Source: CAD feature listing. Evaluate the final solid. Frame: model axes, mm. Give positions to 0.01 mm unless a question says otherwise; leave off trailing zeros. Order: outer loops, then holes, each group sorted by start corner. A loop starts at its lowest first (then second) coordinate and runs counter-clockwise, first axis right, second up. Notation, with made-up numbers: M 43,74.5 L 100,74.5 A23 cw 100,85.5 Z; hole C -35.75,37 d7. An arc over 180 degrees is marked long. Use CSV: the item, a comma, the result in double quotes. Start each with the question number.
1. Pin query (flat end, axial travel): P1, Ø1, axis at x = -47, z = 1, coming from the +Y side; P2, Ø0.6, axis at x = -41.5, z = 1, coming from the -Y side. Return the tip coordinate at first contact, or that it passes through.
2. Section query C-C, the plane y = -3. Return the cut outline in (x, z), plus the area to 3 significant figures.
3. Line query: line 1 along Y through (x, z) = (1, 1.2); line 2 along X through (y, z) = (4.5, 0.85); line 3 along Y through (x, z) = (-22.5, 1.85). Output: solid intervals per line, ascending. Write a range as [from, to].
4. Section query A-A, the plane x = -2. Return the cut outline in (y, z), plus the area to 3 significant figures.
5. Section query D-D, the plane x = 40. Return the cut outline in (y, z), plus the area to 3 significant figures.
6. Section query B-B, the plane y = 15.5. Return the cut outline in (x, z).
from build123d import *

# Parameters (mm, degrees)
F0_R     = 1.5
F0_R_2   = 2.03
F0_W     = 15
F0_H     = 8.7
F1_DEPTH = 2


with BuildPart() as f1:
    # F0 (on Top) → F1 (new body)
    with BuildSketch(Plane.XY):
        Polygon((41.615864, -42.761541), (46.897838, -42.761541), (46.897838, 23.388459), (30.897838, 23.388459), (30.897838, 47.388459), (4.397838, 47.388459), (4.397838, 41.317214), (-8.602162, 41.317214), (-8.602162, 47.388459), (-35.102162, 47.388459), (-35.102162, 23.388459), (-51.102162, 23.388459), (-51.102162, -42.761541), (-45.820188, -42.761541), (-45.820188, -36.761541), (-33.020188, -36.761541), (-33.020188, -42.761541), (28.815864, -42.761541), (28.815864, -36.761541), (41.615864, -36.761541), align=None)
        with Locations((-26.002162, -32.761541)):
            Circle(F0_R, mode=Mode.SUBTRACT)
        with Locations((-27.493694, -8.936541)):
            Circle(F0_R_2, mode=Mode.SUBTRACT)
        with Locations((21.797838, -32.761541)):
            Circle(F0_R, mode=Mode.SUBTRACT)
        with Locations((-1.243694, -0.936335)):
            Rectangle(F0_W, F0_H, mode=Mode.SUBTRACT)
        with Locations((22.506306, -7.686541)):
            Circle(F0_R_2, mode=Mode.SUBTRACT)
        Polygon((-21.34608, 10.93288), (-10.739479, 0.326279), (-16.891308, -5.82555), (-27.497909, 4.781051), align=None, mode=Mode.SUBTRACT)
        with Locations((-17.493694, 22.238665)):
            Circle(F0_R_2, mode=Mode.SUBTRACT)
        with Locations((-31.402162, 24.888459)):
            Circle(F0_R, mode=Mode.SUBTRACT)
        with Locations((-31.402162, 44.888459)):
            Circle(F0_R, mode=Mode.SUBTRACT)
        with Locations((-22.402162, 44.888459)):
            Circle(F0_R, mode=Mode.SUBTRACT)
        Polygon((14.40392, -5.82555), (8.252091, 0.326279), (8.252091, 19.263665), (18.858692, 19.263665), (18.858692, 10.93288), (25.010521, 4.781051), align=None, mode=Mode.SUBTRACT)
        with Locations((15.006306, 22.238665)):
            Circle(F0_R_2, mode=Mode.SUBTRACT)
        with Locations((18.197838, 44.888459)):
            Circle(F0_R, mode=Mode.SUBTRACT)
        with Locations((27.197838, 24.888459)):
            Circle(F0_R, mode=Mode.SUBTRACT)
        with Locations((27.197838, 44.888459)):
            Circle(F0_R, mode=Mode.SUBTRACT)
    extrude(amount=F1_DEPTH)


solid = f1.part
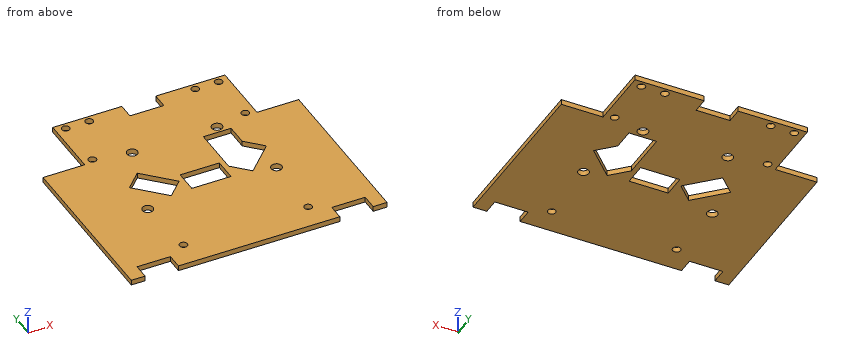
Result set:
1,P1,"y = 23.39"
1,P2,"y = -36.76"
2,outline,"M -51.1,0 L -19.72,0 L -19.72,2 L -51.1,2 Z; M -14.07,0 L -8.74,0 L -8.74,2 L -14.07,2 Z; M 6.26,0 L 11.58,0 L 11.58,2 L 6.26,2 Z; M 17.23,0 L 46.9,0 L 46.9,2 L 17.23,2 Z"
2,area,"143 mm2"
3,line 1,"[-42.76, -5.29], [3.41, 41.32]"
3,line 2,"[-51.1, -27.22], [-14.91, 8.25], [24.73, 46.9]"
3,line 3,"[-42.76, -0.22], [9.78, 43.39], [46.39, 47.39]"
4,outline,"M -42.76,0 L -5.29,0 L -5.29,2 L -42.76,2 Z; M 3.41,0 L 41.32,0 L 41.32,2 L 3.41,2 Z"
4,area,"151 mm2"
5,outline,"M -36.76,0 L 23.39,0 L 23.39,2 L -36.76,2 Z"
5,area,"120 mm2"
6,outline,"M -51.1,0 L 8.25,0 L 8.25,2 L -51.1,2 Z; M 18.86,0 L 46.9,0 L 46.9,2 L 18.86,2 Z"
